from build123d import *

# Parameters (mm, degrees)
SKETCH1_R           = 1.98755
BOSS_EXTRUDE1_DEPTH = 1.524
BOSS_EXTRUDE2_START = -2.4765
SKETCH3_R           = 1.98755
BOSS_EXTRUDE2_DEPTH = 8.27405


with BuildPart() as part:
    # Sketch1 → Boss-Extrude1 (new body)
    with BuildSketch(Plane.XY):
        with BuildLine():
            Line((-12.7, 5.6515), (12.7, 5.6515))
            ThreePointArc((12.7, 5.6515), (18.3515, 0), (12.7, -5.6515))
            Line((12.7, -5.6515), (-12.7, -5.6515))
            ThreePointArc((-12.7, -5.6515), (-18.3515, 0), (-12.7, 5.6515))
        make_face()
        with Locations((-12.7, 0)):
            Circle(SKETCH1_R, mode=Mode.SUBTRACT)
        with Locations((12.7, 0)):
            Circle(SKETCH1_R, mode=Mode.SUBTRACT)
    boss_extrude1 = extrude(amount=BOSS_EXTRUDE1_DEPTH)

    # Sketch3 → Boss-Extrude2 (add)
    with BuildSketch(Plane(origin=(0, 0, 0), x_dir=(-1, 0, 0), z_dir=(0, 0, -1)).offset(BOSS_EXTRUDE2_START)):
        with Locations((-12.7, 0)):
            Circle(SKETCH3_R)
        with Locations((12.7, 0)):
            Circle(SKETCH3_R)
    boss_extrude2 = extrude(amount=BOSS_EXTRUDE2_DEPTH)

    # Mirror4: Boss-Extrude1, Boss-Extrude2 across plane
    add(boss_extrude1.mirror(Plane.XY.offset(-5.79755)))
    add(boss_extrude2.mirror(Plane.XY.offset(-5.79755)))


solid = part.part
Work out the finished part from the listing and answer in its coordinate system (mm). A direction names the side the tool comes from. Round coordinates to 2 decimals unless told otherwise and drop trailing zeros. Write each loop counter-clockwise with the first axis right and the second up, starting at its lowest first coordinate (ties: lowest second). Pieces come first, ordered by that corner, then holes. Notation, with made-up numbers: (-21.5, 56) - (1.5, 56) arc R23 ccw to (1.5, 67) - close; hole circle Ø3 at (45.25, -21). An arc over 180 degrees is marked (long way). Answer in a Markdown table with one row per item. Add a question column.
1. A cutting plane is placed at A-A, the plane x = -4.5. Determine the outline of the cut face in (y, z).
2. A cutting plane is placed at C-C, the plane z = -7. Determine the outline of the cut face in (x, y), and give its area (3 significant figures).
3. Find the intervals of material crossed by line 1 along Z through (x, y) = (-1.5, 2.25); line 2 along X through (y, z) = (-0.25, -11.75); line 3 along X through (y, z) = (-0.25, -1), in increasing order. Write a range as from..to.
4. Given pin 1 (6 mm diameter, centred on y = -2.5, z = -8.5, fed in from -X); pin 2 (5 mm diameter, centred on x = 5.5, z = -11.5, fed in from +Y); pin 3 (5.5 mm diameter, centred on x = -4.5, y = -1, fed in from +Z); pin 4 (1.5 mm diameter, centred on x = 12.5, z = -3.5, fed in from +Y), each flat-ended and moving along its own axis, determine where each tip first touches the part or whether it passes through.
5. The mould has two halves that part along X. Classify faces 4 (the cylindrical face through (18.35, 0.12, -12.35)), 5 (the flat face through (-13, 0, -14.072)), 6 (the flat face through (0, 0, 1.524)): +X half, -X half, draft (parallel to the pull), parting line (faces both ways), or undercut.
6. For faces 1 (the cylindrical face through (14.686, 0.087, -13.602)), 2 (the cylindrical face through (-14.536, -0.761, 2.007)), 3 (the flat face through (13, 0, -14.072)), determine the directions among +Z, -Z, +X, -X, +Y, -Y from which every point of the face is accessible in a straight line to the end or side of a thin tool.
7. A cutting plane is placed at D-D, the plane y = -4.5. Determine the outline of the cut face in (x, z), and give its area (3 significant figures).
Worked out:
| question | item | result |
|---|---|---|
| 1 | outline | (-5.65, -13.12) - (5.65, -13.12) - (5.65, -11.6) - (-5.65, -11.6) - close; (-5.65, 0) - (5.65, 0) - (5.65, 1.52) - (-5.65, 1.52) - close |
| 2 | outline | circle Ø3.98 at (-12.7, 0); circle Ø3.98 at (12.7, 0) |
| 2 | area | 24.8 mm^2 |
| 3 | line 1 | -13.12..-11.6, 0..1.52 |
| 3 | line 2 | -18.35..18.35 |
| 3 | line 3 | -14.67..-10.73, 10.73..14.67 |
| 4 | pin 1 | x = -14.69 |
| 4 | pin 2 | y = 5.65 |
| 4 | pin 3 | z = 1.52 |
| 4 | pin 4 | y = 1.99 |
| 5 | face 4 | +X half |
| 5 | face 5 | draft |
| 5 | face 6 | undercut |
| 6 | face 1 | -Z |
| 6 | face 2 | +Z |
| 6 | face 3 | -Z, +X, -X, +Y, -Y |
| 7 | outline | (-16.12, -13.12) - (16.12, -13.12) - (16.12, -11.6) - (-16.12, -11.6) - close; (-16.12, 0) - (16.12, 0) - (16.12, 1.52) - (-16.12, 1.52) - close |
| 7 | area | 98.3 mm^2 |
